from build123d import *

# Parameters (mm, degrees)
SKETCH1_W           = 25.4
SKETCH1_H           = 25.4
SKETCH1_W_2         = 22.225
SKETCH1_H_2         = 22.225
BOSS_EXTRUDE1_DEPTH = 762
SKETCH3_R           = 2.54
CUT_EXTRUDE2_DEPTH  = 763.846196818
CUT_EXTRUDE3_REACH  = 764.846
SKETCH4_R           = 2.003399785
SKETCH4_R_2         = 2.54
CUT_EXTRUDE4_REACH  = 764.846
SKETCH5_R           = 2.54


with BuildPart() as part:
    # Sketch1 → Boss-Extrude1 (new body)
    with BuildSketch(Plane.XY):
        with Locations((12.7, 12.7)):
            Rectangle(SKETCH1_W, SKETCH1_H)
        with Locations((12.7, 12.7)):
            Rectangle(SKETCH1_W_2, SKETCH1_H_2, mode=Mode.SUBTRACT)
    extrude(amount=BOSS_EXTRUDE1_DEPTH)

    # Sketch3 → Cut-Extrude2 (cut, through all)
    with BuildSketch(Plane(origin=(0, 25.4, 0), x_dir=(1, 0, 0), z_dir=(0, 1, 0))):
        with Locations(Location((12.7, -12.7, 0), (0, 0, 270))):
            Circle(SKETCH3_R)
        with Locations(Location((12.7, -38.1, 0), (0, 0, 270))):
            Circle(SKETCH3_R)
        with Locations(Location((12.7, -723.9, 0), (0, 0, 90))):
            Circle(SKETCH3_R)
        with Locations(Location((12.7, -749.3, 0), (0, 0, 90))):
            Circle(SKETCH3_R)
    extrude(amount=-CUT_EXTRUDE2_DEPTH, mode=Mode.SUBTRACT)

    # Sketch4 → Cut-Extrude3 (cut, up to next)
    with BuildSketch(Plane(origin=(25.4, 0, 0), x_dir=(0, 0, -1), z_dir=(1, 0, 0)), mode=Mode.PRIVATE) as cut_extrude3_sk1:
        with Locations((-6.35, 12.7)):
            Circle(SKETCH4_R)
    cut_extrude3_tool1 = extrude(cut_extrude3_sk1.sketch, amount=-CUT_EXTRUDE3_REACH, mode=Mode.PRIVATE) & part.part
    # Sketch4 → Cut-Extrude3 (cut, up to next)
    with BuildSketch(Plane(origin=(25.4, 0, 0), x_dir=(0, 0, -1), z_dir=(1, 0, 0)), mode=Mode.PRIVATE) as cut_extrude3_sk2:
        with Locations((-31.75, 12.7)):
            Circle(SKETCH4_R_2)
    cut_extrude3_tool2 = extrude(cut_extrude3_sk2.sketch, amount=-CUT_EXTRUDE3_REACH, mode=Mode.PRIVATE) & part.part
    add(cut_extrude3_tool1.solids().sort_by_distance((25.4, 12.7, 6.35))[0], mode=Mode.SUBTRACT)
    add(cut_extrude3_tool2.solids().sort_by_distance((25.4, 12.7, 31.75))[0], mode=Mode.SUBTRACT)

    # Sketch5 → Cut-Extrude4 (cut, up to next)
    with BuildSketch(Plane.ZY, mode=Mode.PRIVATE) as cut_extrude4_sk1:
        with Locations((39.6875, 12.7)):
            Circle(SKETCH5_R)
    cut_extrude4_tool1 = extrude(cut_extrude4_sk1.sketch, amount=-CUT_EXTRUDE4_REACH, mode=Mode.PRIVATE) & part.part
    # Sketch5 → Cut-Extrude4 (cut, up to next)
    with BuildSketch(Plane.ZY, mode=Mode.PRIVATE) as cut_extrude4_sk2:
        with Locations((722.3125, 12.7)):
            Circle(SKETCH5_R)
    cut_extrude4_tool2 = extrude(cut_extrude4_sk2.sketch, amount=-CUT_EXTRUDE4_REACH, mode=Mode.PRIVATE) & part.part
    add(cut_extrude4_tool1.solids().sort_by_distance((0, 12.7, 39.6875))[0], mode=Mode.SUBTRACT)
    add(cut_extrude4_tool2.solids().sort_by_distance((0, 12.7, 722.3125))[0], mode=Mode.SUBTRACT)


solid = part.part
Here's how the part is built. I have some questions about the finished solid (model axes, mm). A direction names the side the tool comes from. Coordinates: 2 decimals unless noted, no trailing zeros. Loops run counter-clockwise (first coordinate to the right, second up) from the corner with the lowest first, then second, coordinate; pieces in that order, holes last. Notation, with made-up numbers: (20.5, 52.5) -> (69.5, 52.5) arc R23 cw to (69.5, 76.5) -> close; hole circle Ø7 at (21.5, 69.5). An arc over 180 degrees is marked (long way). Use one line per item in the form item = value. Start each with the question number.
(1) We'd pull the mould along Y, two halves only. Please class faces 3 (the face through (13, 25.4, 376)), 4 (the face through (23.812, 13, 376)), 5 (the face through (13, 0, 376)): pulls with the +Y half, pulls with the -Y half, needs draft (parallel to the pull), parting line crosses it, or undercut.
(2) If we section it at A-A (z = 170.5): Please give me the cut outline in (x, y), then the cut area to 3 significant figures.
(3) Please list where these lines run through material, in increasing order: line 1 along Y through (x, z) = (21.5, 229.5); line 2 along Y through (x, z) = (24.2, 31.75).
(4) On a 3-axis mill with a long thin cutter (end or side, diameter ignored), from which of +Z, -Z, +X, -X, +Y, -Y can I reach the whole of each face in a straight line? I mean faces 1 (the face through (1, 13, 0)), 2 (the face through (1.587, 13, 376)). Say none if no direction works.
(5) Will these pins go through, and if not, where does the flat tip stop? pin 1 (8 mm diameter, centred on x = 6.5, y = 18, fed in from +Z); pin 2 (3.5 mm diameter, centred on y = 12.7, z = 6.35, fed in from +X).
Verdict:
q1.face_3 = pulls with the +Y half
q1.face_4 = undercut
q1.face_5 = pulls with the -Y half
q2.outline = (0, 0) -> (25.4, 0) -> (25.4, 25.4) -> (0, 25.4) -> close; hole (1.59, 1.59) -> (23.81, 1.59) -> (23.81, 23.81) -> (1.59, 23.81) -> close
q2.area = 151 mm²
q3.line_1 = 0 to 1.59, 23.81 to 25.4
q3.line_2 = 0 to 10.16, 15.24 to 25.4
q4.face_1 = -Z, +X, -X, +Y, -Y
q4.face_2 = +Z, -Z
q5.pin_1 = through
q5.pin_2 = 1.59
